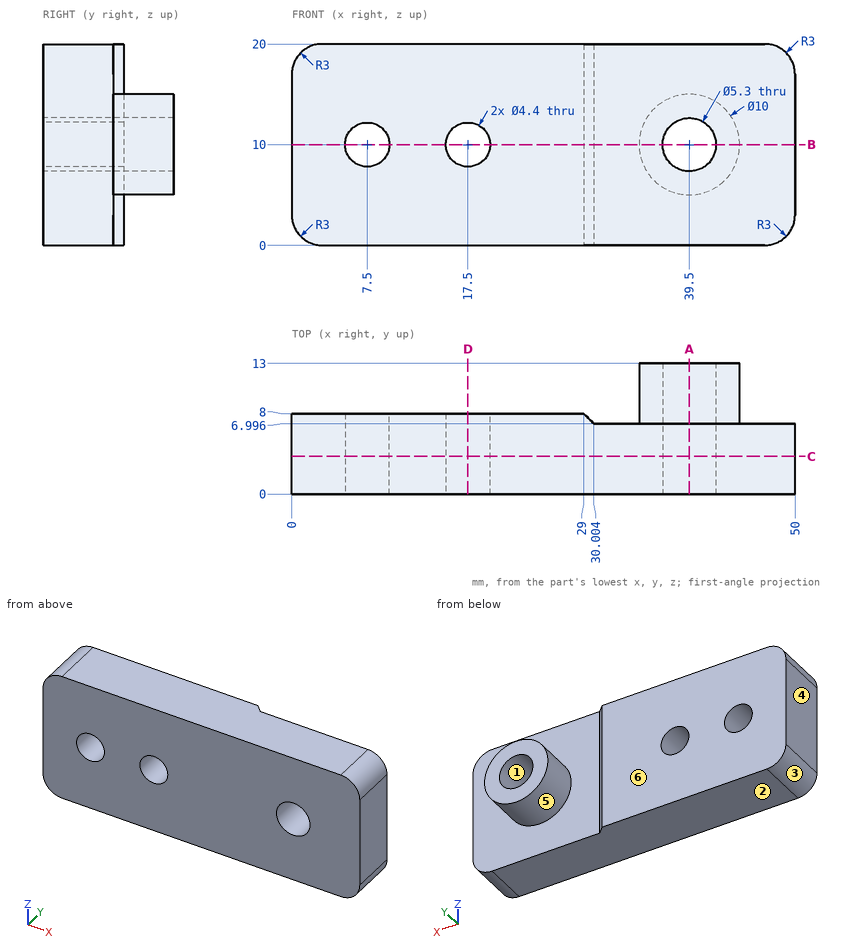
The drawing under review shows one solid part. Ordinate dimensions are in mm from its lowest x, y, z. A direction names the side the tool comes from. Coordinates: 2 decimals unless noted, no trailing zeros. Order: outer loops, then holes, each group sorted by start corner. A loop starts at its lowest first (then second) coordinate and runs counter-clockwise, first axis right, second up. Notation, with made-up numbers: M 45.5,64.25 L 103.5,64.25 A20 ccw 103.5,103.25 Z; hole C 14,40 d11. An arc over 180 degrees is marked long. Use a Markdown table: item, result.
(1) For P1, Ø5, axis at x = 39.5, z = 10, coming from the +Y side; P2, Ø2, axis at y = 11.5, z = 5.5, coming from the +X side; P3, Ø1.5, axis at y = 11, z = 11.5, coming from the -X side, all flat-tipped, find the tip position at first contact; note any pin that passes through.
Worked answers:
| item | result |
|---|---|
| P1 | passes through |
| P2 | stops at x = 43.07 |
| P3 | stops at x = 34.56 |
(2) Add section B-B (z = 10). Give the boundary of the cut face in (x, y).
Worked answers:
| item | result |
|---|---|
| outline | M 0,0 L 5.3,0 L 5.3,8 L 0,8 Z; M 9.7,0 L 15.3,0 L 15.3,8 L 9.7,8 Z; M 19.7,0 L 36.85,0 L 36.85,13 L 34.5,13 L 34.5,7 L 30,7 L 29,8 L 19.7,8 Z; M 42.15,0 L 50,0 L 50,7 L 44.5,7 L 44.5,13 L 42.15,13 Z |
(3) Add section C-C (y = 3.75). Give the boundary of the cut face in (x, z), then the cut area to 3 significant figures.
Worked answers:
| item | result |
|---|---|
| outline | M 0,3 A3 ccw 3,0 L 47,0 A3 ccw 50,3 L 50,17 A3 ccw 47,20 L 3,20 A3 ccw 0,17 Z; hole C 7.5,10 d4.4; hole C 17.5,10 d4.4; hole C 39.5,10 d5.3 |
| area | 940 mm2 |
(4) Draft analysis for pull direction X (two halves, no side actions). For the marked faces 1, 2 and 3, state which applies: released by +X, released by -X, zero draft, split by the parting line, or undercut.
Worked answers:
| item | result |
|---|---|
| face 1 | undercut |
| face 2 | zero draft |
| face 3 | released by -X |
(5) For the marked faces 4, 5 and 6, list the 3-axis set-ups (+Z, -Z, +X, -X, +Y, -Y) from which the entire face can be reached by the end or side of a thin tool; tool diameter is ignored.
Worked answers:
| item | result |
|---|---|
| face 4 | +Z, -Z, -X, +Y, -Y |
| face 5 | +Y |
| face 6 | +Z, -Z, -X, +Y |
(6) Add section D-D (x = 17.5). Give the boundary of the cut face in (y, z).
Worked answers:
| item | result |
|---|---|
| outline | M 0,0 L 8,0 L 8,7.8 L 0,7.8 Z; M 0,12.2 L 8,12.2 L 8,20 L 0,20 Z |
(7) Add section A-A (x = 39.5). Give the boundary of the cut face in (y, z).
Worked answers:
| item | result |
|---|---|
| outline | M 0,0 L 7,0 L 7,5 L 13,5 L 13,7.35 L 0,7.35 Z; M 0,12.65 L 13,12.65 L 13,15 L 7,15 L 7,20 L 0,20 Z |
(8) Wall thickness on probe 1 along Z at (x, y) = (39.5, 6.5); probe 2 along Z at (x, y) = (39.5, 9.5); probe 3 along X at (y, z) = (2.25, 11.5) (1 decimal): over which ranges is each line inside the solid? List them lowest first.
Worked answers:
| item | result |
|---|---|
| probe 1 | z = 0 to 7.35, 12.65 to 20 |
| probe 2 | z = 5 to 7.35, 12.65 to 15 |
| probe 3 | x = 0 to 5.9, 9.1 to 15.9, 19.1 to 37.3, 41.7 to 50 |
